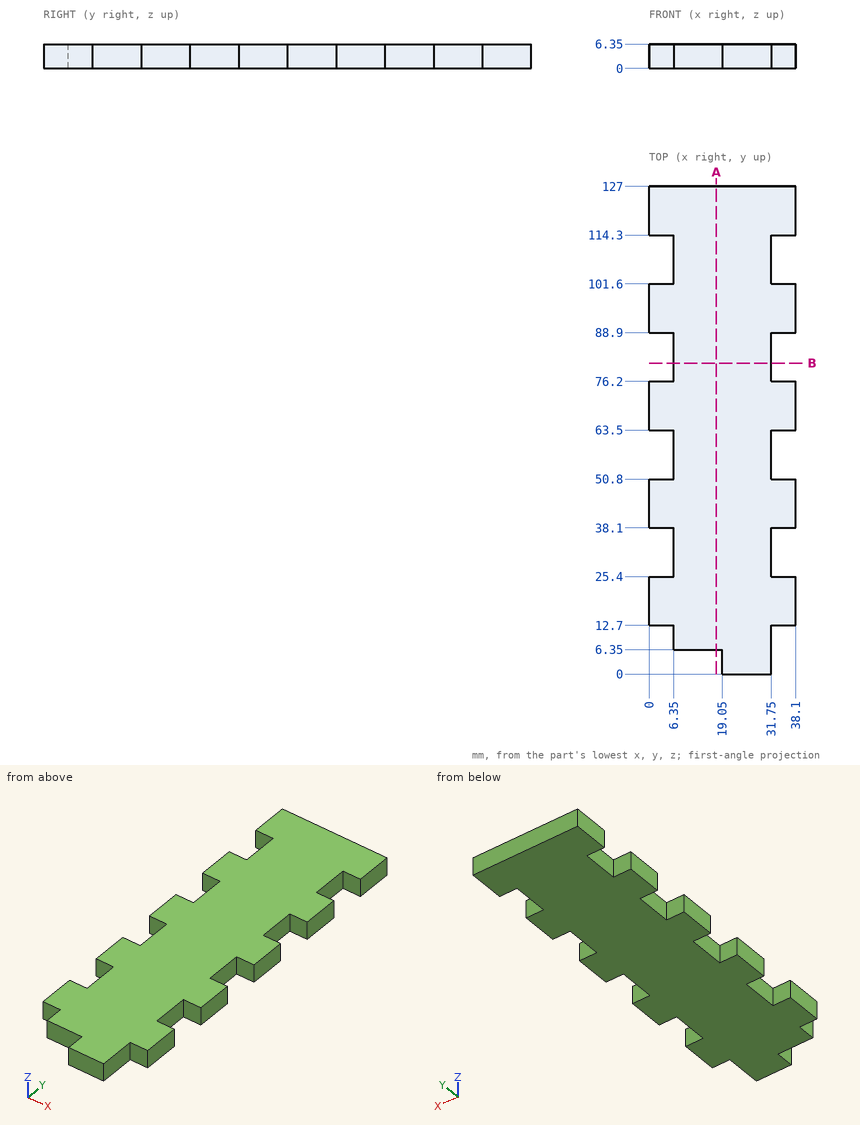
For this review, use the dimensioned drawing (mm, ordinates from the lowest corner) and the shaded views. Round coordinates to 2 decimals unless told otherwise and drop trailing zeros. Write each loop counter-clockwise with the first axis right and the second up, starting at its lowest first coordinate (ties: lowest second). Pieces come first, ordered by that corner, then holes. Notation, with made-up numbers: M -33.5,25 L -0.5,25 A33 cw -0.5,59 Z; hole C 44.5,3.5 d9. An arc over 180 degrees is marked long. Write item = value, one per line. Start each with the question number.
(1) We need section B-B (y = 81). Give the boundary of the cut face in (x, z).
(2) We need section A-A (x = 17.5). Give the boundary of the cut face in (y, z), then the cut area to 3 significant figures.
(3) For line 1 along Y through (x, z) = (36, 2.5); line 2 along X through (y, z) = (79.5, 1.5); line 3 along Y through (x, z) = (15.5, 0.5), list the stretches that pass through material, from the lowest coordinate up.
(4) Clearance check with flat-ended pins moving along their axes: pin 1 Ø1.9 at (y, z) = (109, 4) entering from -X; pin 2 Ø1.9 at (x, z) = (3, 3) entering from -Y; pin 3 Ø1.9 at (y, z) = (105.5, 4.5) entering from +X. State where each tip first meets the part, or that it passes through.
Results found:
q1.outline = M 6.35,0 L 31.75,0 L 31.75,6.35 L 6.35,6.35 Z
q2.outline = M 6.35,0 L 127,0 L 127,6.35 L 6.35,6.35 Z
q2.area = 766 mm²
q3.line_1 = 12.7 to 25.4, 38.1 to 50.8, 63.5 to 76.2, 88.9 to 101.6, 114.3 to 127
q3.line_2 = 6.35 to 31.75
q3.line_3 = 6.35 to 127
q4.pin_1 = 6.35
q4.pin_2 = 12.7
q4.pin_3 = 31.75
